```python
from build123d import *

# Parameters (mm, degrees)
EXT_BODY_DEPTH          = 1.55
CUT_POT_HOLE_DEPTH      = 15.946906034
CUT_POT_HOLE_DEPTH_BACK = 15.946906034
SKETCH2_R               = 2
SKETCH5_R               = 0.15
EXT_PINS_DEPTH          = 3.4


with BuildPart() as part:
    # Sketch1 → ext-body (new, symmetric)
    with BuildSketch(Plane.XY):
        with BuildLine():
            Line((0.75, 0), (8.65, 0))
            ThreePointArc((8.65, 0), (9.180330086, 0.219669914), (9.4, 0.75))
            Line((9.4, 0.75), (9.4, 10.45))
            ThreePointArc((9.4, 10.45), (9.180330086, 10.980330086), (8.65, 11.2))
            Line((8.65, 11.2), (0.75, 11.2))
            ThreePointArc((0.75, 11.2), (0.219669914, 10.980330086), (0, 10.45))
            Line((0, 10.45), (0, 0.75))
            ThreePointArc((0, 0.75), (0.219669914, 0.219669914), (0.75, 0))
        make_face()
    extrude(amount=EXT_BODY_DEPTH, both=True)

    # Sketch2 → cut-pot_hole (cut, two sides: drawn at the far end of the back side and taken through both)
    with BuildSketch(Plane.XY.offset(1.55).offset(-CUT_POT_HOLE_DEPTH_BACK)):
        with Locations((4.7, 6.5)):
            Circle(SKETCH2_R)
    extrude(amount=CUT_POT_HOLE_DEPTH + CUT_POT_HOLE_DEPTH_BACK, mode=Mode.SUBTRACT)

    # Sketch5 → ext-pins (add)
    with BuildSketch(Plane.XZ):
        with Locations(Location((2.35, 0, 0), (0, 0, 90))):
            Circle(SKETCH5_R)
        with Locations(Location((4.7, 0, 0), (0, 0, 90))):
            Circle(SKETCH5_R)
        with Locations(Location((7.05, 0, 0), (0, 0, 90))):
            Circle(SKETCH5_R)
    extrude(amount=EXT_PINS_DEPTH)


solid = part.part
```
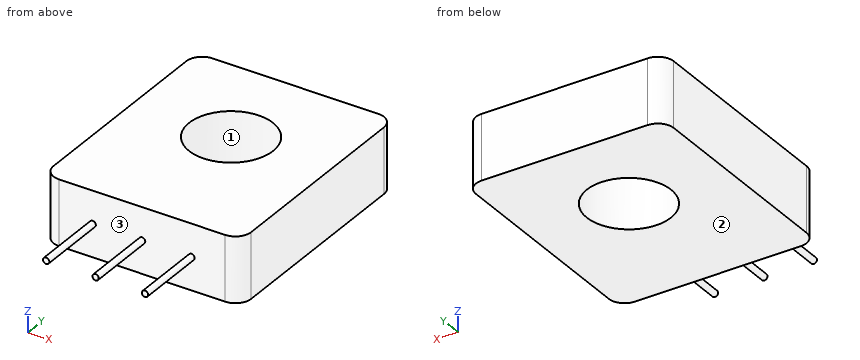
Could you check a few things on this model? Use its own coordinates, in mm. Face numbers are marked on the shaded views. Round coordinates to 2 decimals unless told otherwise and drop trailing zeros. Loops run counter-clockwise (first coordinate to the right, second up) from the corner with the lowest first, then second, coordinate; pieces in that order, holes last. Notation, with made-up numbers: M 50.25,7.25 L 95.25,7.25 A22 cw 95.25,32.25 Z; hole C 72.25,43 d4. An arc over 180 degrees is marked long. Write item = value, one per line.
1. I want a section at C-C, the plane x = 3.25. Write out the boundary of the cut face in (y, z), and give its area (3 significant figures).
Results below:
outline = M 0,-1.55 L 5.12,-1.55 L 5.12,1.55 L 0,1.55 Z; M 7.88,-1.55 L 11.2,-1.55 L 11.2,1.55 L 7.88,1.55 Z
area = 26.2 mm²
2. I want a section at B-B, the plane z = 0. Write out the boundary of the cut face in (x, y), and give its area (3 significant figures).
Results below:
outline = M 0,0.75 A0.75 ccw 0.75,0 L 2.2,0 L 2.2,-3.4 L 2.5,-3.4 L 2.5,0 L 4.55,0 L 4.55,-3.4 L 4.85,-3.4 L 4.85,0 L 6.9,0 L 6.9,-3.4 L 7.2,-3.4 L 7.2,0 L 8.65,0 A0.75 ccw 9.4,0.75 L 9.4,10.45 A0.75 ccw 8.65,11.2 L 0.75,11.2 A0.75 ccw 0,10.45 Z; hole C 4.7,6.5 d4
area = 95.3 mm²
3. I want a section at A-A, the plane y = 6.5. Write out the boundary of the cut face in (x, z), and give its area (3 significant figures).
Results below:
outline = M 0,-1.55 L 2.7,-1.55 L 2.7,1.55 L 0,1.55 Z; M 6.7,-1.55 L 9.4,-1.55 L 9.4,1.55 L 6.7,1.55 Z
area = 16.7 mm²
4. I need wall thicknesses on probe 1 along X at (y, z) = (6.5, -0.15); probe 2 along Y at (x, z) = (4.7, -0.9); probe 3 along Y at (x, z) = (4.75, -0.1). Which ranges of each line are inside material? Lowest first, please.
Results below:
probe_1 = 0 to 2.7, 6.7 to 9.4
probe_2 = 0 to 4.5, 8.5 to 11.2
probe_3 = -3.4 to 4.5, 8.5 to 11.2
5. I want a section at D-D, the plane y = -1.5. Write out the boundary of the cut face in (x, z), and give its area (3 significant figures).
Results below:
outline = C 2.35,0 d0.3; C 4.7,0 d0.3; C 7.05,0 d0.3
area = 0.212 mm²
6. Thinking about a two-plate mould opening in Y: for the marked faces 1, 2 and 3, which applies, +Y half, -Y half, draft (parallel to the pull), parting line (faces both ways), or undercut?
Results below:
face_1 = undercut
face_2 = draft
face_3 = -Y half
